Check sheet for the drawn part. Datum: minimum x, y, z corner. Units: mm. A direction names the side the tool comes from. Coordinates: 2 decimals unless noted, no trailing zeros. Write each loop counter-clockwise with the first axis right and the second up, starting at its lowest first coordinate (ties: lowest second). Pieces come first, ordered by that corner, then holes. Notation, with made-up numbers: M 22.5,1.5 L 53.5,1.5 A36 cw 53.5,36.5 Z; hole C 29.5,61.5 d8. An arc over 180 degrees is marked long. Answer as CSV lines item,"result".
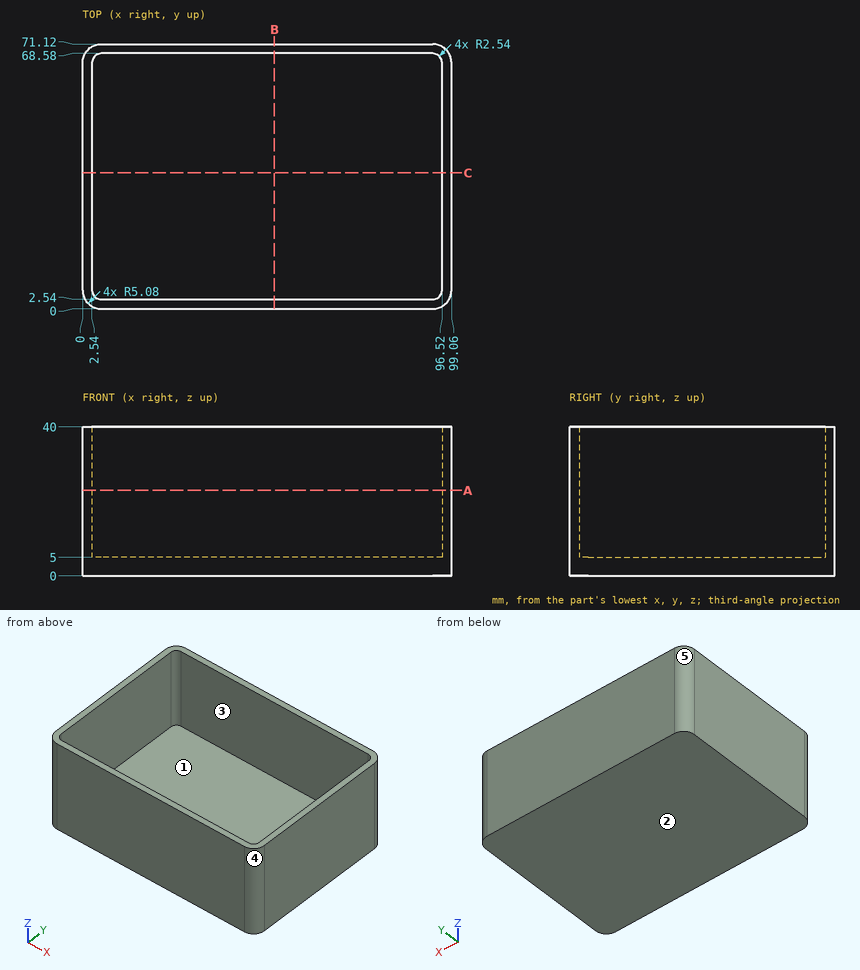
1) Section check A-A, the plane z = 23. Record the boundary of the cut face in (x, y).
Answer key:
outline,"M 0,5.08 A5.08 ccw 5.08,0 L 93.98,0 A5.08 ccw 99.06,5.08 L 99.06,66.04 A5.08 ccw 93.98,71.12 L 5.08,71.12 A5.08 ccw 0,66.04 Z; hole M 2.54,5.08 A2.54 ccw 5.08,2.54 L 93.98,2.54 A2.54 ccw 96.52,5.08 L 96.52,66.04 A2.54 ccw 93.98,68.58 L 5.08,68.58 A2.54 ccw 2.54,66.04 Z"
2) Depth check by flat-ended pin: P1, Ø8, axis at x = 73, y = 18.5, coming from the +Z side. Enter the tip coordinate at first touch or a pass-through.
Answer key:
P1,"stops at z = 5"
3) Tool access check on the marked faces 1 and 2. Record the directions out of +Z, -Z, +X, -X, +Y, -Y that give a thin tool (end or side, any length) a straight path to the whole face; none if there is none.
Answer key:
face 1,"+Z"
face 2,"-Z, +X, -X, +Y, -Y"
4) Thickness scan on line 1 along Y through (x, z) = (90, 22); line 2 along X through (y, z) = (7.5, 29); line 3 along Z through (x, y) = (33, 28). Record the ranges inside material, lowest first.
Answer key:
line 1,"y = 0 to 2.54, 68.58 to 71.12"
line 2,"x = 0 to 2.54, 96.52 to 99.06"
line 3,"z = 0 to 5"
5) Section check C-C, the plane y = 36.5. Record the boundary of the cut face in (x, z), plus the area to 3 significant figures.
Answer key:
outline,"M 0,0 L 99.06,0 L 99.06,40 L 96.52,40 L 96.52,5 L 2.54,5 L 2.54,40 L 0,40 Z"
area,"673 mm2"
6) Mould release check, pull along Y, two halves, no side actions. Record for the marked faces 3, 4 and 5: pulls with the +Y half, pulls with the -Y half, needs draft (parallel to the pull), parting line crosses it, or undercut.
Answer key:
face 3,"undercut"
face 4,"pulls with the -Y half"
face 5,"pulls with the +Y half"
7) Section check B-B, the plane x = 51.5. Record the boundary of the cut face in (y, z).
Answer key:
outline,"M 0,0 L 71.12,0 L 71.12,40 L 68.58,40 L 68.58,5 L 2.54,5 L 2.54,40 L 0,40 Z"
